Can you work these out from the model? Positions are in its coordinate system, mm. Give positions to 0.01 mm unless a question says otherwise; leave off trailing zeros. Loops run counter-clockwise (first coordinate to the right, second up) from the corner with the lowest first, then second, coordinate; pieces in that order, holes last. Notation, with made-up numbers: (25.25, 65) - (56.25, 65) arc R22 cw to (56.25, 78) - close; hole circle Ø7 at (3, -35.5). An arc over 180 degrees is marked (long way). Use a Markdown table: item, result. Add a question column.
```python
from build123d import *

# Parameters (mm, degrees)
SKETCH1_W           = 140
SKETCH1_H           = 30
BOSS_EXTRUDE1_DEPTH = 3
SKETCH2_R           = 1
SKETCH2_W           = 23
SKETCH2_H           = 12
CUT_EXTRUDE1_DEPTH  = 4
FILLET1_R           = 14


with BuildPart() as part:
    # Sketch1 → Boss-Extrude1 (new body)
    with BuildSketch(Plane(origin=(0, 0, 0), x_dir=(1, 0, 0), z_dir=(0, 1, 0))):
        with Locations((70, 15)):
            Rectangle(SKETCH1_W, SKETCH1_H)
    extrude(amount=BOSS_EXTRUDE1_DEPTH)

    # Sketch2 → Cut-Extrude1 (cut, through all)
    with BuildSketch(Plane(origin=(0, 3, 0), x_dir=(1, 0, 0), z_dir=(0, 1, 0))):
        with Locations((20, 15)):
            Circle(SKETCH2_R)
        with Locations((114.5, 15)):
            Rectangle(SKETCH2_W, SKETCH2_H)
    extrude(amount=-CUT_EXTRUDE1_DEPTH, mode=Mode.SUBTRACT)

    # Fillet1
    fillet1_edges = [part.edges().sort_by_distance(p)[0] for p in [
        (0, 1.5, -30),
        (140, 1.5, -30),
        (140, 1.5, 0),
        (0, 1.5, 0),
    ]]
    fillet(fillet1_edges, radius=FILLET1_R)


solid = part.part
```
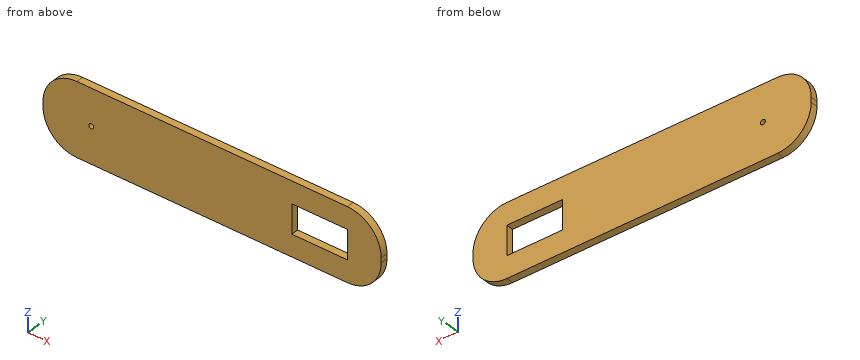
1. Suppose I cut it at B-B (y = 0.65). List the corners of the cut face in (x, z) for me, and give its area (3 significant figures).
2. Suppose I cut it at C-C (z = -19). List the corners of the cut face in (x, y) for me.
3. Please list where these lines run through material, in increasing order: line 1 along X through (y, z) = (2, -15); line 2 along Z through (x, y) = (20, 1.05); line 3 along X through (y, z) = (2.85, -13.25). Write a range as [from, to].
4. Suppose I cut it at D-D (z = -28). List the corners of the cut face in (x, y) for me.
5. Suppose I cut it at A-A (x = 111). List the corners of the cut face in (y, z) for me, and give its area (3 significant figures).
Results below:
| question | item | result |
|---|---|---|
| 1 | outline | (0, -16) arc R14 ccw to (14, -30) - (126, -30) arc R14 ccw to (140, -16) - (140, -14) arc R14 ccw to (126, 0) - (14, 0) arc R14 ccw to (0, -14) - close; hole circle Ø2 at (20, -15); hole (103, -21) - (126, -21) - (126, -9) - (103, -9) - close |
| 1 | area | 3,750 mm² |
| 2 | outline | (0.33, 0) - (103, 0) - (103, 3) - (0.33, 3) - close; (126, 0) - (139.67, 0) - (139.67, 3) - (126, 3) - close |
| 3 | line 1 | [0, 19], [21, 103], [126, 140] |
| 3 | line 2 | [-30, -16], [-14, 0] |
| 3 | line 3 | [0.02, 103], [126, 139.98] |
| 4 | outline | (6.79, 0) - (133.21, 0) - (133.21, 3) - (6.79, 3) - close |
| 5 | outline | (0, -30) - (3, -30) - (3, -21) - (0, -21) - close; (0, -9) - (3, -9) - (3, 0) - (0, 0) - close |
| 5 | area | 54.0 mm² |
